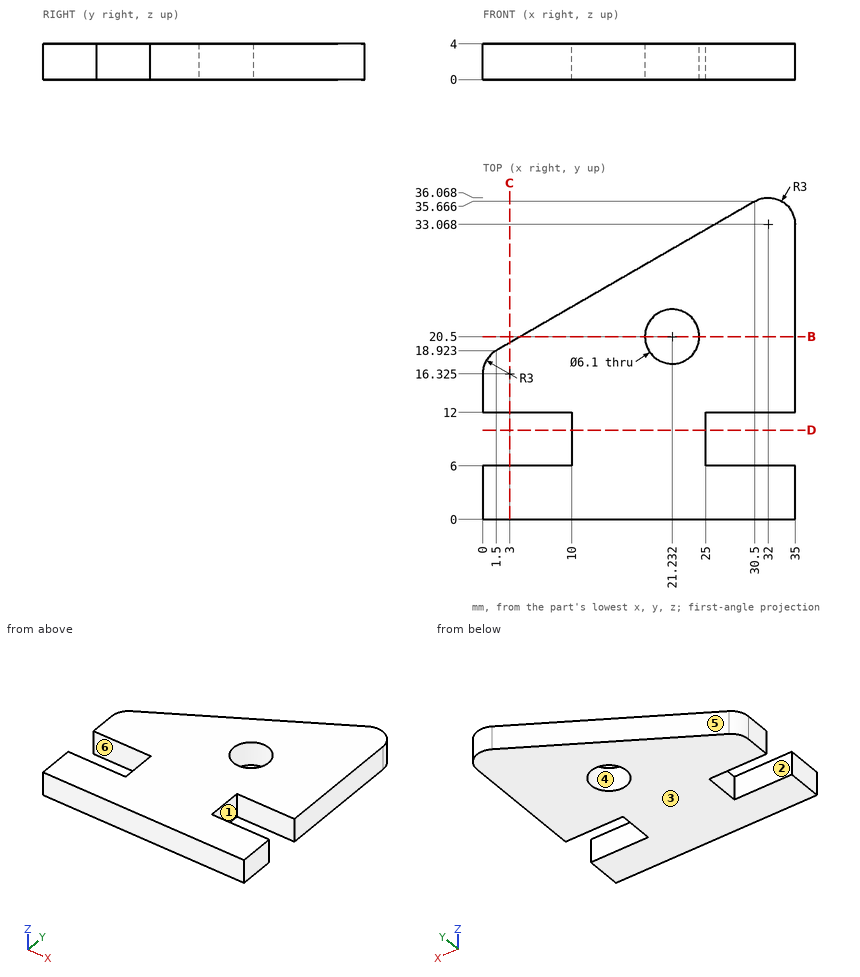
Print and shaded views of the part. All mm, measured from the part's lowest x, y and z. A direction names the side the tool comes from. Coordinates: 2 decimals unless noted, no trailing zeros. Order: outer loops, then holes, each group sorted by start corner. A loop starts at its lowest first (then second) coordinate and runs counter-clockwise, first axis right, second up. Notation, with made-up numbers: (87, -18) -> (115, -18) arc R27 cw to (115, 18) -> close; hole circle Ø5 at (72, -16.5). An arc over 180 degrees is marked (long way). Use one line per item in the form item = value. Start each with the question number.
1) Band-saw the part on C-C on x = 3. Give the cut face in (y, z).
2) Pull direction X, two halves, no side cores. Call the marked faces 4, 5 and 6: +X half, -X half, draft (parallel to the pull), parting line (faces both ways), or undercut.
3) Tool access for the marked faces 1, 2 and 3: list every direction of +Z, -Z, +X, -X, +Y, -Y with a clear straight run to the whole face (end or side of a thin tool).
4) Drop flat-ended pins along their axis: pin 1 (1 mm diameter, centred on y = 29, z = 2.5, fed in from -X); pin 2 (1.5 mm diameter, centred on y = 31.5, z = 2, fed in from -X) (1 decimal); pin 3 (2 mm diameter, centred on x = 30.5, z = 1, fed in from +Y); pin 4 (3.5 mm diameter, centred on x = 21.23, y = 20.5, fed in from +Z). Give the stop position or say it passes through.
5) Band-saw the part on B-B on y = 20.5. Give the cut face in (x, z).
6) Band-saw the part on D-D on y = 10. Give the cut face in (x, z).
7) Drill centre lines: L1, parallel to Y at x = 33.5, z = 0.9 (1 decimal); L2, parallel to X at y = 10, z = 1.8; L3, parallel to Y at x = 28.5, z = 1.25. Where is each one in solid material? Low to high. Write a range as [from, to].
Entries:
q1.outline = (0, 0) -> (6, 0) -> (6, 4) -> (0, 4) -> close; (12, 0) -> (19.79, 0) -> (19.79, 4) -> (12, 4) -> close
q2.face_4 = undercut
q2.face_5 = -X half
q2.face_6 = draft
q3.face_1 = +Z, -Z, +X
q3.face_2 = +Z, -Z, -X
q3.face_3 = -Z, +X, -X, +Y, -Y
q4.pin_1 = 18.09
q4.pin_2 = 22
q4.pin_3 = 36.03
q4.pin_4 = through
q5.outline = (4.23, 0) -> (18.18, 0) -> (18.18, 4) -> (4.23, 4) -> close; (24.28, 0) -> (35, 0) -> (35, 4) -> (24.28, 4) -> close
q6.outline = (10, 0) -> (25, 0) -> (25, 4) -> (10, 4) -> close
q7.L1 = [0, 6], [12, 35.7]
q7.L2 = [10, 25]
q7.L3 = [0, 6], [12, 34.51]
